Could you check a few things on this model? Use its own coordinates, in mm. A direction names the side the tool comes from. Coordinates: 2 decimals unless noted, no trailing zeros. Order: outer loops, then holes, each group sorted by start corner. A loop starts at its lowest first (then second) coordinate and runs counter-clockwise, first axis right, second up. Notation, with made-up numbers: (-6, 32.5) - (6, 32.5) arc R32 cw to (6, 68.5) - close; hole circle Ø11 at (18.25, 71). An arc over 180 degrees is marked (long way). Answer as CSV lines item,"result". Start each with the question number.
1. Thinking about a two-plate mould opening in X: for faces 1 (the face through (13, 0, 3)), 2 (the face through (25.4, 3, 3)), 3 (the face through (63.5, 28, 3)), which applies, released by +X, released by -X, zero draft, split by the parting line, or undercut?
2. I want a section at A-A, the plane z = 2.95. List the corners of the cut face in (x, y) for me, and give its area (3 significant figures).
3. I want a section at B-B, the plane x = 22.5. List the corners of the cut face in (y, z) for me, and give its area (3 significant figures).
4. For faces 4 (the face through (19, 25.4, 3)), 5 (the face through (88.9, 28, 3)), 6 (the face through (45, 19, 0)), which set-ups out of +Z, -Z, +X, -X, +Y, -Y let a thin tool reach every point of the face, with its end or its side?
5. I need wall thicknesses on probe 1 along X at (y, z) = (28.5, 0.4); probe 2 along Y at (x, z) = (15, 0.55). Which ranges of each line are inside material? Lowest first, please.
6. For pin 1 (1.6 mm diameter, centred on y = 3.5, z = 3.5, fed in from +X); pin 2 (1.6 mm diameter, centred on y = 28.5, z = 3, fed in from -X); pin 3 (1 mm diameter, centred on x = 64, y = 14.5, fed in from -Z); pin 4 (2 mm diameter, centred on x = 13.5, z = 4, fed in from +Y), each with a flat end and sliding along its axis, tell me the tip position at first contact or that it passes through.
from build123d import *

# Parameters (mm, degrees)
BOSS_EXTRUDE1_DEPTH = 5.461
FILLET1_R           = 2.54


with BuildPart() as part:
    # Sketch1 → Boss-Extrude1 (new body)
    with BuildSketch(Plane.XY):
        Polygon((0, 0), (0, 25.4), (38.1, 25.4), (38.1, 30.988), (63.5, 30.988), (63.5, 25.4), (88.9, 25.4), (88.9, 30.988), (114.3, 30.988), (114.3, 25.4), (114.3, 19.05), (25.4, 5.588), (25.4, 0), align=None)
    extrude(amount=BOSS_EXTRUDE1_DEPTH)

    # Fillet1
    fillet1_edges = [part.edges().sort_by_distance(p)[0] for p in [
        (114.3, 19.05, 2.7305),
    ]]
    fillet(fillet1_edges, radius=FILLET1_R)


solid = part.part
Solved:
1,face 1,"zero draft"
1,face 2,"released by +X"
1,face 3,"undercut"
2,outline,"(0, 0) - (25.4, 0) - (25.4, 5.59) - (112.14, 18.72) arc R2.54 ccw to (114.3, 21.23) - (114.3, 30.99) - (88.9, 30.99) - (88.9, 25.4) - (63.5, 25.4) - (63.5, 30.99) - (38.1, 30.99) - (38.1, 25.4) - (0, 25.4) - close"
2,area,"2,090 mm2"
3,outline,"(0, 0) - (25.4, 0) - (25.4, 5.46) - (0, 5.46) - close"
3,area,"139 mm2"
4,face 4,"+Z, -Z, -X, +Y"
4,face 5,"+Z, -Z, +Y"
4,face 6,"-Z, +X, -X, +Y, -Y"
5,probe 1,"x = 38.1 to 63.5, 88.9 to 114.3"
5,probe 2,"y = 0 to 25.4"
6,pin 1,"stops at x = 25.4"
6,pin 2,"stops at x = 38.1"
6,pin 3,"stops at z = 0"
6,pin 4,"stops at y = 25.4"
